Source: CAD feature listing. Evaluate the final solid. Frame: model axes, mm. Face numbers are marked on the shaded views. A direction names the side the tool comes from. Coordinates: 2 decimals unless noted, no trailing zeros. Write each loop counter-clockwise with the first axis right and the second up, starting at its lowest first coordinate (ties: lowest second). Pieces come first, ordered by that corner, then holes. Notation, with made-up numbers: (25, 79.25) -> (42, 79.25) arc R13 ccw to (42, 98.25) -> close; hole circle Ø7 at (-14, -2). An arc over 180 degrees is marked (long way). Write item = value, one per line.
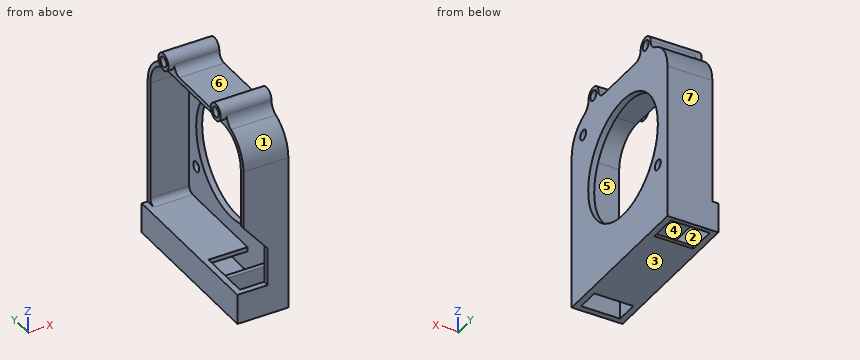
from build123d import *

# Parameters (mm, degrees)
PAD014_DEPTH    = 17
POCKET010_DEPTH = 15
SKETCH035_R     = 1.7
SKETCH035_R_2   = 20
POCKET011_DEPTH = 17
SKETCH036_W     = 0.5
SKETCH036_H     = 10.1
PAD015_DEPTH    = 13
SKETCH037_W     = 52
SKETCH037_H     = 10.1
PAD016_DEPTH    = 2
SKETCH038_W     = 53.5
SKETCH038_H     = 2
POCKET012_DEPTH = 55
POCKET013_DEPTH = 2
POCKET014_DEPTH = 1.5


with BuildPart() as part:
    # Sketch033 → Pad014 (new body)
    with BuildSketch(Plane.YZ):
        with BuildLine():
            Line((27.5, -61.35), (-27.5, -61.35))
            Line((-27.5, -51.25), (-27.5, -61.35))
            Line((-27.5, -9.2536580703), (-27.5, -51.25))
            ThreePointArc((-20.3403225806, 1.3958301754), (-25.5436814091, -2.837417336), (-27.5, -9.2536580703))
            ThreePointArc((-20.3403225806, 1.3958301754), (-18.5304586403, 2.8682640924), (-17.85, 5.1))
            ThreePointArc((-12.15, 5.1), (-15, 7.95), (-17.85, 5.1))
            ThreePointArc((-12.15, 5.1), (-11.3152543264, 3.0847456736), (-9.3, 2.25))
            Line((-9.3, 2.25), (9.3, 2.25))
            ThreePointArc((9.3, 2.25), (11.3152543264, 3.0847456736), (12.15, 5.1))
            ThreePointArc((17.85, 5.1), (15, 7.95), (12.15, 5.1))
            ThreePointArc((17.85, 5.1), (18.5304586403, 2.8682640924), (20.3403225806, 1.3958301754))
            ThreePointArc((27.5, -9.2536580703), (25.5436814091, -2.837417336), (20.3403225806, 1.3958301754))
            Line((27.5, -9.2536580703), (27.5, -51.25))
            Line((27.5, -51.25), (27.5, -61.35))
        make_face()
    extrude(amount=-PAD014_DEPTH)

    # Sketch034 (on Face16 of Pad014) → Pocket010 (cut)
    with BuildSketch(Plane(origin=(-17, 0, 0), x_dir=(0, -1, 0), z_dir=(-1, 0, 0))):
        with BuildLine():
            Line((26, -9.2536580703), (26, -61.35))
            Line((-26, -61.35), (26, -61.35))
            Line((-26, -61.35), (-26, -9.2536580703))
            ThreePointArc((-16, 0.7463419297), (-23.0710678119, -2.1825902585), (-26, -9.2536580703))
            Line((16, 0.7463419297), (-16, 0.7463419297))
            ThreePointArc((26, -9.2536580703), (23.0710678119, -2.1825902585), (16, 0.7463419297))
        make_face()
    extrude(amount=-POCKET010_DEPTH, mode=Mode.SUBTRACT)

    # Sketch035 (on Face4 of Pocket010) → Pocket011 (cut)
    with BuildSketch(Plane.YZ):
        with Locations((-15, 5.1)):
            Circle(SKETCH035_R)
        with Locations((15, 5.1)):
            Circle(SKETCH035_R)
        with Locations((-20.9, -5.25)):
            Circle(SKETCH035_R)
        with Locations((2, -26.25)):
            Circle(SKETCH035_R_2)
        with Locations((21.982166, -40.391422)):
            Circle(SKETCH035_R)
    extrude(amount=-POCKET011_DEPTH, mode=Mode.SUBTRACT)

    # Sketch036 (on Face27 of Pocket011) → Pad015 (join)
    with BuildSketch(Plane(origin=(-2, 0, 0), x_dir=(0, -1, 0), z_dir=(-1, 0, 0))):
        with BuildLine():
            ThreePointArc((17.9, -51.85), (17.3390474824, -51.2512719364), (16.7050823529, -51.7720705882))
            ThreePointArc((7.5, -59.85), (13.623448471, -57.5441622111), (16.7050823529, -51.7720705882))
            Line((7.5, -59.85), (-15.5, -59.85))
            ThreePointArc((-15.5, -59.85), (-16.2071067812, -60.1428932188), (-16.5, -60.85))
            Line((-16.5, -60.85), (-16.5, -61.35))
            Line((17.9, -61.35), (-16.5, -61.35))
            Line((17.9, -51.85), (17.9, -61.35))
        make_face()
        with Locations((25.75, -56.3)):
            Rectangle(SKETCH036_W, SKETCH036_H)
        with BuildLine():
            Line((-26, -49.25), (-26, -55.75))
            ThreePointArc((-23, -52.75), (-25.1213203436, -53.6286796564), (-26, -55.75))
            Line((7.5, -52.75), (-23, -52.75))
            Line((7.5, -51.25), (7.5, -52.75))
            Line((7.5, -51.25), (-24, -51.25))
            ThreePointArc((-26, -49.25), (-25.4142135624, -50.6642135624), (-24, -51.25))
        make_face()
    extrude(amount=PAD015_DEPTH)

    # Sketch037 (on Face31 of Pad015) → Pad016 (join)
    with BuildSketch(Plane(origin=(-15, 0, 0), x_dir=(0, -1, 0), z_dir=(-1, 0, 0))):
        with Locations((0, -56.3)):
            Rectangle(SKETCH037_W, SKETCH037_H)
    extrude(amount=PAD016_DEPTH)

    # Sketch038 (on Face11 of Pad016) → Pocket012 (cut)
    with BuildSketch(Plane(origin=(0, -27.5, 0), x_dir=(0, 0, 1), z_dir=(0, -1, 0))):
        with Locations((-24.5, 16)):
            Rectangle(SKETCH038_W, SKETCH038_H)
    extrude(amount=-POCKET012_DEPTH, mode=Mode.SUBTRACT)

    # Sketch039 (on Face33 of Pocket012) → Pocket013 (cut)
    with BuildSketch(Plane(origin=(-17, 0, 0), x_dir=(0, -1, 0), z_dir=(-1, 0, 0))):
        with BuildLine():
            ThreePointArc((-17.85, 5.1), (-15, 2.25), (-12.15, 5.1))
            Line((-9.3, 5.1), (-12.15, 5.1))
            Line((-9.3, 5.1), (-9.3, 0))
            Line((-9.3, 0), (-19.0433115599, 0))
            Line((-19.0433115599, 0), (-19.0433115599, 5.1))
            Line((-17.85, 5.1), (-19.0433115599, 5.1))
        make_face()
        with BuildLine():
            ThreePointArc((12.15, 5.1), (15, 2.25), (17.85, 5.1))
            Line((17.85, 5.1), (19.0433115599, 5.1))
            Line((19.0433115599, 5.1), (19.0433115599, 0))
            Line((19.0433115599, 0), (9.3, 0))
            Line((9.3, 0), (9.3, 5.1))
            Line((9.3, 5.1), (12.15, 5.1))
        make_face()
    extrude(amount=-POCKET013_DEPTH, mode=Mode.SUBTRACT)

    # Sketch040 (on Face11 of Pocket013) → Pocket014 (cut)
    with BuildSketch(Plane(origin=(0, -27.5, 0), x_dir=(0, 0, 1), z_dir=(0, -1, 0))):
        Polygon((-51.25, 15), (-51.25, 7), (-38.3735294118, 7), (-28.7264705882, 15), align=None)
    extrude(amount=-POCKET014_DEPTH, mode=Mode.SUBTRACT)


with BuildPart() as part_1:
    # Body006 placement: moved
    add(part.part.moved(Location((35, 0, 0))))


solid = part_1.part
1) Cut plane B-B, the plane y = 2. Output: boundary loops of the cut face in (x, z).
Answer block:
outline = (18, -61.35) -> (35, -61.35) -> (35, -46.25) -> (33, -46.25) -> (33, -51.25) -> (18, -51.25) -> close; (20, 0.75) -> (33, 0.75) -> (33, -6.25) -> (35, -6.25) -> (35, 2.25) -> (20, 2.25) -> close; hole (20, -59.85) -> (33, -59.85) -> (33, -52.75) -> (20, -52.75) -> close
2) Cut plane A-A, the plane x = 19. Output: boundary loops of the cut face in (y, z).
Answer block:
outline = (-27.5, -61.35) -> (27.5, -61.35) -> (27.5, -51.25) -> (-27.5, -51.25) -> close; circle Ø5.7 at (-15, 5.1); circle Ø5.7 at (15, 5.1); hole circle Ø3.4 at (-15, 5.1); hole circle Ø3.4 at (15, 5.1)
3) Material intervals for probe 1 along Z at (x, y) = (29.5, 15); probe 2 along Y at (x, z) = (32.25, -37); probe 3 along Z at (x, y) = (20.25, -2.5), sorted ascending. Write a range as [from, to].
Answer block:
probe_1 = [-61.35, -59.85], [-52.75, -51.25], [0.75, 3.4], [6.8, 7.95]
probe_2 = [-27.5, -26], [26, 27.5]
probe_3 = [-61.35, -59.85], [-52.75, -51.25], [0.75, 2.25]
4) Cut plane D-D, the plane z = -44. Output: boundary loops of the cut face in (x, y).
Answer block:
outline = (20, 26) -> (33, 26) -> (33, 11.22) -> (35, 11.22) -> (35, 27.5) -> (20, 27.5) -> close; (28, -27.5) -> (35, -27.5) -> (35, -7.22) -> (33, -7.22) -> (33, -26) -> (28, -26) -> close
5) First-contact query: pin 1 Ø6.5 at (x, y) = (26, 1.5) entering from +Z; pin 2 Ø4 at (x, y) = (24.5, -19.5) entering from +Z. Flat tips, straight axial feed; report the tip coordinate or a pass-through.
Answer block:
pin_1 = 2.25
pin_2 = 6.47
6) Reachability of the marked faces 4, 5, 6 and 7 from +Z, -Z, +X, -X, +Y, -Y: full face, straight path, thin tool, end or side. Return the list, or none.
Answer block:
face_4 = none
face_5 = -X
face_6 = +Z, +X, -X
face_7 = +Z, -Z, +X, -X, +Y
7) Cut plane C-C, the plane x = 31. Give the number of separate pieces and of enclosed holes in the cut face, and give its area (3 significant figures).
Answer block:
separate_pieces = 2
enclosed_holes = 2
area = 439 mm2
8) Pull-direction query (Z, two-part tool) for the marked faces 1, 2 and 3; classes: +Z half, -Z half, draft (parallel to the pull), parting line (faces both ways), or undercut.
Answer block:
face_1 = +Z half
face_2 = undercut
face_3 = -Z half
